```python
from build123d import *

# Parameters (mm, degrees)
BOSS_EXTRUDE1_DEPTH                      = 62.5
BOSS_EXTRUDE2_REACH                      = 273.512
CUT_EXTRUDE1_DEPTH                       = 229.538281314
FILLET1_R                                = 20
SKETCH6_R                                = 10
CUT_EXTRUDE2_DEPTH                       = 267.134431621
CUT_EXTRUDE3_DEPTH                       = 10
CBORE_FOR_M24_HEX_HEAD_BOLT1_D           = 26
CBORE_FOR_M24_HEX_HEAD_BOLT1_CBORE_D     = 44.569
CBORE_FOR_M24_HEX_HEAD_BOLT1_CBORE_DEPTH = 15
CUT_EXTRUDE4_START                       = 165
SKETCH6_3_R                              = 10
CUT_EXTRUDE4_DEPTH                       = 101.814175539
BOSS_EXTRUDE4_DEPTH                      = 7


with BuildPart() as part:
    # Sketch1 → Boss-Extrude1 (new, symmetric)
    with BuildSketch(Plane.XY):
        Polygon((190, 150), (190, 65), (0, 65), (0, 0), (-25, 0), (-25, 90), (165, 90), (165, 150), align=None)
    extrude(amount=BOSS_EXTRUDE1_DEPTH, both=True)

    # Sketch4 → Boss-Extrude2 (add, up to next)
    with BuildSketch(Plane(origin=(-57.5, 57.5, 0), x_dir=(0.7071067811865475, 0.7071067811865477, 0), z_dir=(0.7071067811865477, -0.7071067811865475, 0)), mode=Mode.PRIVATE) as boss_extrude2_sk1:
        with BuildLine():
            Line((45.961940777, -36), (130.961940777, -36))
            ThreePointArc((130.961940777, -36), (166.961940777, 0), (130.961940777, 36))
            Line((130.961940777, 36), (45.961940777, 36))
            Line((45.961940777, 36), (45.961940777, -36))
        make_face()
    boss_extrude2_tool1 = extrude(boss_extrude2_sk1.sketch, amount=BOSS_EXTRUDE2_REACH, mode=Mode.PRIVATE) - part.part
    add(boss_extrude2_tool1.solids().sort_by_distance((15.250037, 130.250037, 0))[0])

    # Sketch5 → Cut-Extrude1 (cut, through all)
    with BuildSketch(Plane(origin=(0, 65, 0), x_dir=(-1, 0, 0), z_dir=(0, -1, 0))):
        with BuildLine():
            Line((-125, -47.5), (-25, -47.5))
            ThreePointArc((-25, -47.5), (-14.393398282, -73.106601718), (-40, -62.5))
            Line((-40, -62.5), (-110, -62.5))
            ThreePointArc((-110, -62.5), (-135.606601718, -73.106601718), (-125, -47.5))
        make_face()
        with BuildLine():
            Line((-125, 47.5), (-25, 47.5))
            ThreePointArc((-25, 47.5), (-14.393398282, 73.106601718), (-40, 62.5))
            Line((-40, 62.5), (-110, 62.5))
            ThreePointArc((-110, 62.5), (-135.606601718, 73.106601718), (-125, 47.5))
        make_face()
    extrude(amount=-CUT_EXTRUDE1_DEPTH, mode=Mode.SUBTRACT)

    # Fillet1
    fillet1_edges = [part.edges().sort_by_distance(p)[0] for p in [
        (177.5, 150, -62.5),
        (-12.5, 0, 62.5),
        (177.5, 150, 62.5),
        (-12.5, 0, -62.5),
    ]]
    fillet(fillet1_edges, radius=FILLET1_R)

    # Sketch6 → Cut-Extrude2 (cut, through all)
    with BuildSketch(Plane(origin=(0, 0, 0), x_dir=(0, 0, -1), z_dir=(1, 0, 0))):
        with Locations((42.5, 20)):
            Circle(SKETCH6_R)
        with Locations((-42.5, 20)):
            Circle(SKETCH6_R)
    extrude(amount=-CUT_EXTRUDE2_DEPTH, mode=Mode.SUBTRACT)

    # Sketch7 → Cut-Extrude3 (cut)
    with BuildSketch(Plane(origin=(-57.5, 57.5, 0), x_dir=(0, 0, 1), z_dir=(-0.7071067811865438, 0.7071067811865513, 0))):
        with BuildLine():
            Line((-7, 166.274827943), (-7, 27.494892071))
            Line((-7, 27.494892071), (7, 27.494892071))
            Line((7, 27.494892071), (7, 166.274827943))
            ThreePointArc((7, 166.274827943), (0, 166.961940777), (-7, 166.274827943))
        make_face()
    extrude(amount=-CUT_EXTRUDE3_DEPTH, mode=Mode.SUBTRACT)

    # CBORE for M24 Hex Head Bolt1 (through all)
    with Locations(Plane(origin=(-57.5, 57.5, 0), x_dir=(0, 0, 1), z_dir=(-0.7071067811865438, 0.7071067811865513, 0))):
        with Locations((0, 130.961940777)):
            CounterBoreHole(CBORE_FOR_M24_HEX_HEAD_BOLT1_D / 2, CBORE_FOR_M24_HEX_HEAD_BOLT1_CBORE_D / 2, CBORE_FOR_M24_HEX_HEAD_BOLT1_CBORE_DEPTH)

    # Sketch6<3> → Cut-Extrude4 (cut, through all)
    with BuildSketch(Plane(origin=(0, 0, 0), x_dir=(0, 0, -1), z_dir=(1, 0, 0)).offset(CUT_EXTRUDE4_START)):
        with Locations((42.5, 20)):
            Circle(SKETCH6_3_R)
        with Locations((-42.5, 20)):
            Circle(SKETCH6_3_R)
        with Locations((42.5, 130)):
            Circle(SKETCH6_3_R)
        with Locations((-42.5, 130)):
            Circle(SKETCH6_3_R)
    extrude(amount=CUT_EXTRUDE4_DEPTH, mode=Mode.SUBTRACT)

    # Sketch11 → Boss-Extrude4 (add, symmetric)
    with BuildSketch(Plane.XY):
        Polygon((165, 130), (97.583974217, 130), (137.512677947, 90), (165, 90), align=None)
    extrude(amount=BOSS_EXTRUDE4_DEPTH, both=True)


solid = part.part
```
Design review of the part built by this model. Coordinates are the model's own, in mm. A direction names the side the tool comes from. Give positions to 0.01 mm unless a question says otherwise; leave off trailing zeros. Loops run counter-clockwise (first coordinate to the right, second up) from the corner with the lowest first, then second, coordinate; pieces in that order, holes last. Notation, with made-up numbers: M -39.5,48.5 L 10.5,48.5 A25 cw 10.5,72.5 Z; hole C -20,51 d1. An arc over 180 degrees is marked long. Return JSON: item names as keys, results as strings. Group by question number.
Item 1: Mouldability with a two-part tool opening along Z and no side actions: class faces 6 (the cylindrical face through (-12.32, 26.76, 49.87)), 7 (the flat face through (-11, 55, 62.5)), 8 (the flat face through (76, 77, -47.5)) as released by +Z, released by -Z, zero draft, split by the parting line, or undercut.
Item 2: We need section C-C (y = 49). Give the boundary of the cut face in (x, z), and give its area (4 significant figures).
Item 3: We need section A-A (y = 12.5). Give the boundary of the cut face in (x, z).
Item 4: Tool access review of faces 1 (the flat face through (96, 65, 1)), 2 (the flat face through (-3, 105, 7)), 3 (the flat face through (35, 104, 36)), 4 (the flat face through (177, 150, 1)), 5 (the flat face through (34, 117, -36)): name each direction out of +Z, -Z, +X, -X, +Y, -Y from which nothing blocks a thin tool from reaching the whole face with its end or side.
Item 5: We need section B-B (x = -7). Give the boundary of the cut face in (y, z).
Item 6: Insertion check: pin 1 Ø2 at (x, y) = (97.5, 96) entering from -Z; pin 2 Ø5 at (x, y) = (56, 167) entering from -Z; pin 3 Ø20 at (x, y) = (78, 83.5) entering from -Z. Each pin has a flat end and moves straight along its axis. Give the tip position at first contact, or say it passes through.
Item 7: For probe 1 along Y at (x, z) = (174, -42); probe 2 along Z at (x, y) = (171.25, 130); probe 3 along Y at (x, z) = (-9.25, 42.5), list the stretches that pass through material, from the lowest coordinate up.
Output:
{
 "1": {"face 6": "undercut", "face 7": "released by +Z", "face 8": "released by -Z"},
 "2": {"outline": "M -25,-62.5 L 0,-62.5 L 0,62.5 L -25,62.5 Z", "area": "3,125 mm^2"},
 "3": {"outline": "M -25,-61.04 L 0,-61.04 L 0,-49.11 L -25,-49.11 Z; M -25,-35.89 L 0,-35.89 L 0,35.89 L -25,35.89 Z; M -25,49.11 L 0,49.11 L 0,61.04 L -25,61.04 Z"},
 "4": {"face 1": "+Z, -Z, +X, -Y", "face 2": "-X, +Y", "face 3": "+Z, -X, +Y", "face 4": "+Z, -Z, +X, +Y", "face 5": "-Z, -X, +Y"},
 "5": {"outline": "M 0,-42.5 A20 ccw 20,-62.5 L 90,-62.5 L 90,-36 L 108,-36 L 108,-7 L 93.86,-7 L 93.86,7 L 108,7 L 108,36 L 90,36 L 90,62.5 L 20,62.5 A20 ccw 0,42.5 Z; hole C 20,-42.5 d20; hole C 20,42.5 d20"},
 "6": {"pin 1": "stops at z = -35.67", "pin 2": "stops at z = -26.63", "pin 3": "stops at z = -47.5"},
 "7": {"probe 1": "y = 65 to 120.01, 139.99 to 150", "probe 2": "z = -62.5 to -52.5, -32.5 to 32.5, 52.5 to 62.5", "probe 3": "y = 0 to 10, 30 to 90"}
}
